The model under review builds one solid part; all positions refer to its coordinate system, in mm. A direction names the side the tool comes from. Coordinates: 2 decimals unless noted, no trailing zeros. Loops run counter-clockwise (first coordinate to the right, second up) from the corner with the lowest first, then second, coordinate; pieces in that order, holes last. Notation, with made-up numbers: (47.5, 75) - (88.5, 75) arc R22 ccw to (88.5, 86) - close; hole circle Ø9 at (67, -1). An arc over 180 degrees is marked (long way). Answer in a Markdown table with one row per item. Add a question column.
(1) We need section B-B on x = 7.75. Write out the cut boundary in (y, z) (3 decimals).
(2) For line 1 along Y through (x, z) = (9, 77); line 2 along Y through (x, z) = (-2.25, 24); line 3 along Z through (x, y) = (4.75, -40), list the stretches that pass through material, from the lowest coordinate up.
(3) Machinability: for faces 1 (the cylindrical face through (-1.37, -7.18, 21.06)), 2 (the flat face through (3.46, -45.93, 80.91)), 3 (the flat face through (3, 4.064, 4)), 4 (the flat face through (3.456, -49.29, 73.507)), which of the approach directions +Z, -Z, +X, -X, +Y, -Y give a long, thin tool a straight path to every point of the face, cutting with its end or side? Answer none if there is none.
(4) Mouldability with a two-part tool opening along Y and no side actions: class faces 5 (the flat face through (-2.983, -31, 37)), 6 (the flat face through (3.46, -46.12, 90.9)), 7 (the cylindrical face through (3.456, -34.546, 71.206)), 8 (the cylindrical face through (-1.417, 7.046, 21.648)) as +Y half, -Y half, draft (parallel to the pull), parting line (faces both ways), or undercut.
(5) We need section A-A on y = 38. Write out the cut boundary in (x, z).
(6) For P1, Ø11.5, axis at y = 40.26, z = 73.97, coming from the -X side; P2, Ø5, axis at x = 6, z = 5.5, coming from the -Y side; P3, Ø5, axis at x = 6.5, z = 26, coming from the -Y side; P4, Ø3, axis at x = 5, z = 3, coming from the +Y side, all flat-tipped, find the tip position at first contact; note any pin that passes through.
(7) We need section C-C on y = -36. Write out the cut boundary in (x, z) (3 decimals).
from build123d import *

# Parameters (mm, degrees)
F4_DEPTH  = 12.7
F5_SIZE   = 1.016
F8_W      = 3.175
F8_H      = 6.35
F12_DEPTH = 12.7
F13_SIZE  = 1.016


with BuildPart() as f2:
    # F2: sweep along a path in F1
    with BuildLine(Plane.YZ) as f2_path:
        ThreePointArc((0, 0), (-13.9895526568, 47.0829736144), (-51.4187773904, 78.8881166537))
    # F0 (on Top) → F2 (sweep)
    with BuildSketch(Plane.XY):
        Polygon((-2.9826171882, -15.875), (-2.9826171882, -20.955), (9.7173828118, -20.955), (9.7173828118, 20.955), (-2.9826171882, 20.955), (-2.9826171882, 15.875), (0.1923828118, 15.875), (0.1923828118, 9.525), (-2.9826171882, 9.525), (-2.9826171882, -9.525), (0.1923828118, -9.525), (0.1923828118, -15.875), align=None)
    sweep(path=f2_path.line)

    # F3 (on face) → F4 (cut, through all)
    with BuildSketch(Plane.YZ.offset(9.7173828118)):
        with BuildLine():
            Line((-4.064, 7.3128193311), (-4.064, 0))
            Line((-4.064, 0), (4.064, 0))
            Line((4.064, 0), (4.064, 7.3128193311))
            ThreePointArc((4.064, 7.3128193311), (0, 18.542), (-4.064, 7.3128193311))
        make_face()
        with BuildLine():
            Line((-43.0877289811, 79.6543117793), (-49.7782573242, 82.6062868909))
            Line((-49.7782573242, 82.6062868909), (-53.0592974567, 75.1699464166))
            Line((-53.0592974567, 75.1699464166), (-46.3687691136, 72.217971305))
            ThreePointArc((-46.3687691136, 72.217971305), (-34.4546256835, 71.4032438515), (-43.0877289811, 79.6543117793))
        make_face()
    extrude(amount=-F4_DEPTH, mode=Mode.SUBTRACT)

    # F5
    f5_edges = [f2.edges().sort_by_distance(p)[0] for p in [
        (3.367383, -53.059297, 75.169946),
        (3.367383, -49.778257, 82.606287),
        (3.367383, 4.064, 0),
        (3.367383, -4.064, 0),
    ]]
    chamfer(f5_edges, length=F5_SIZE)

    # F7: sweep along a path in F6
    with BuildLine(Plane.YZ) as f7_path:
        ThreePointArc((51.4187773904, 78.8881166537), (13.9895526568, 47.0829736144), (0, 0))
    # F0 (on Top) → F7 (sweep)
    with BuildSketch(Plane.XY):
        Polygon((-2.9826171882, -15.875), (-2.9826171882, -20.955), (9.7173828118, -20.955), (9.7173828118, 20.955), (-2.9826171882, 20.955), (-2.9826171882, 15.875), (0.1923828118, 15.875), (0.1923828118, 9.525), (-2.9826171882, 9.525), (-2.9826171882, -9.525), (0.1923828118, -9.525), (0.1923828118, -15.875), align=None)
    sweep(path=f7_path.line)

    # F9: sweep along a path in F9_path
    with BuildLine(Plane(origin=(-2.9826171882, 20.955, 0), x_dir=(0, 0, 1), z_dir=(1, 0, 0))) as f9_path:
        ThreePointArc((0, 0), (35.6406156079, -10.5897361719), (59.7163013685, -38.922708982))
    # F8 (on face) → F9 (sweep, cut)
    with BuildSketch(Plane(origin=(0, 0, 0), x_dir=(1, 0, 0), z_dir=(0, 0, -1))):
        with Locations((-1.3951171882, -12.7)):
            Rectangle(F8_W, F8_H)
        with Locations((-1.3951171882, 12.7)):
            Rectangle(F8_W, F8_H)
    sweep(path=f9_path.line, mode=Mode.SUBTRACT)

    # F10: sweep along a path in F10_path
    with BuildLine(Plane(origin=(-2.9826171882, -59.877708982, 59.7163013685), x_dir=(0, 0, 1), z_dir=(1, 0, 0))) as f10_path:
        ThreePointArc((0, 0), (-24.0756857607, -28.33297281), (-59.7163013685, -38.922708982))
    # F8 (on face) → F10 (sweep, cut)
    with BuildSketch(Plane(origin=(0, 0, 0), x_dir=(1, 0, 0), z_dir=(0, 0, -1))):
        with Locations((-1.3951171882, -12.7)):
            Rectangle(F8_W, F8_H)
        with Locations((-1.3951171882, 12.7)):
            Rectangle(F8_W, F8_H)
    sweep(path=f10_path.line, mode=Mode.SUBTRACT)

    # F11 (on face) → F12 (cut, through all)
    with BuildSketch(Plane.YZ.offset(9.7173828118)):
        with BuildLine():
            Line((-4.064, 0), (4.064, 0))
            Line((4.064, 0), (4.064, 7.3128193311))
            ThreePointArc((4.064, 7.3128193311), (0, 18.542), (-4.064, 7.3128193311))
            Line((-4.064, 7.3128193311), (-4.064, 0))
        make_face()
        with BuildLine():
            Line((46.3687691136, 72.217971305), (53.0592974567, 75.1699464166))
            Line((53.0592974567, 75.1699464166), (49.7782573242, 82.6062868909))
            Line((49.7782573242, 82.6062868909), (43.0877289811, 79.6543117793))
            ThreePointArc((43.0877289811, 79.6543117793), (34.4546256835, 71.4032438515), (46.3687691136, 72.217971305))
        make_face()
    extrude(amount=-F12_DEPTH, mode=Mode.SUBTRACT)

    # F13
    f13_edges = [f2.edges().sort_by_distance(p)[0] for p in [
        (3.367383, 4.064, 0),
        (3.367383, -4.064, 0),
        (3.367383, 53.059297, 75.169946),
        (3.367383, 49.778257, 82.606287),
    ]]
    chamfer(f13_edges, length=F13_SIZE)


solid = f2.part
Outcome:
| question | item | result |
|---|---|---|
| 1 | outline | (-59.878, 59.716) arc R65.271 cw to (-20.955, 0) - (-5.08, 0) - (-4.064, 1.016) - (-4.064, 7.313) arc R6.35 cw (long way) to (4.064, 7.313) - (4.064, 1.016) - (5.08, 0) - (20.955, 0) arc R65.271 cw to (59.878, 59.716) - (53.469, 74.24) - (52.13, 74.76) - (46.369, 72.218) arc R6.35 cw (long way) to (43.088, 79.654) - (48.849, 82.196) - (49.368, 83.536) - (42.96, 98.06) arc R107.181 ccw to (0, 63.662) arc R107.181 ccw to (-42.96, 98.06) - (-49.368, 83.536) - (-48.849, 82.196) - (-43.088, 79.654) arc R6.35 cw (long way) to (-46.369, 72.218) - (-52.13, 74.76) - (-53.469, 74.24) - close |
| 2 | line 1 | -34.69 to -11.67, 11.67 to 34.69 |
| 2 | line 2 | -25.53 to -20.1, -13.38 to -13.01, -6.47 to 6.47, 13.01 to 13.38, 20.1 to 25.53 |
| 2 | line 3 | 46.08 to 67.62, 80.31 to 96.7 |
| 3 | face 1 | -X |
| 3 | face 2 | +X, -X, -Y |
| 3 | face 3 | -Z, +X, -X |
| 3 | face 4 | +X, -X |
| 4 | face 5 | draft |
| 4 | face 6 | -Y half |
| 4 | face 7 | undercut |
| 4 | face 8 | undercut |
| 5 | outline | (-2.98, 43.98) - (9.72, 43.98) - (9.72, 68.03) - (-2.98, 68.03) - (-2.98, 59.64) - (0.19, 59.64) - (0.19, 51.22) - (-2.98, 51.22) - close; (-2.98, 79.9) - (9.72, 79.9) - (9.72, 95.72) - (-2.98, 95.72) - (-2.98, 89.99) - (0.19, 89.99) - (0.19, 82.72) - (-2.98, 82.72) - close |
| 6 | P1 | through |
| 6 | P2 | y = -21.45 |
| 6 | P3 | y = -27.51 |
| 6 | P4 | y = 21.11 |
| 7 | outline | (-2.983, 41.685) - (9.717, 41.685) - (9.717, 69.261) - (-2.983, 69.261) - (-2.983, 57.969) - (0.192, 57.969) - (0.192, 49.26) - (-2.983, 49.26) - close; (-2.983, 78.672) - (9.717, 78.672) - (9.717, 94.684) - (-2.983, 94.684) - (-2.983, 88.893) - (0.192, 88.893) - (0.192, 81.52) - (-2.983, 81.52) - close |
